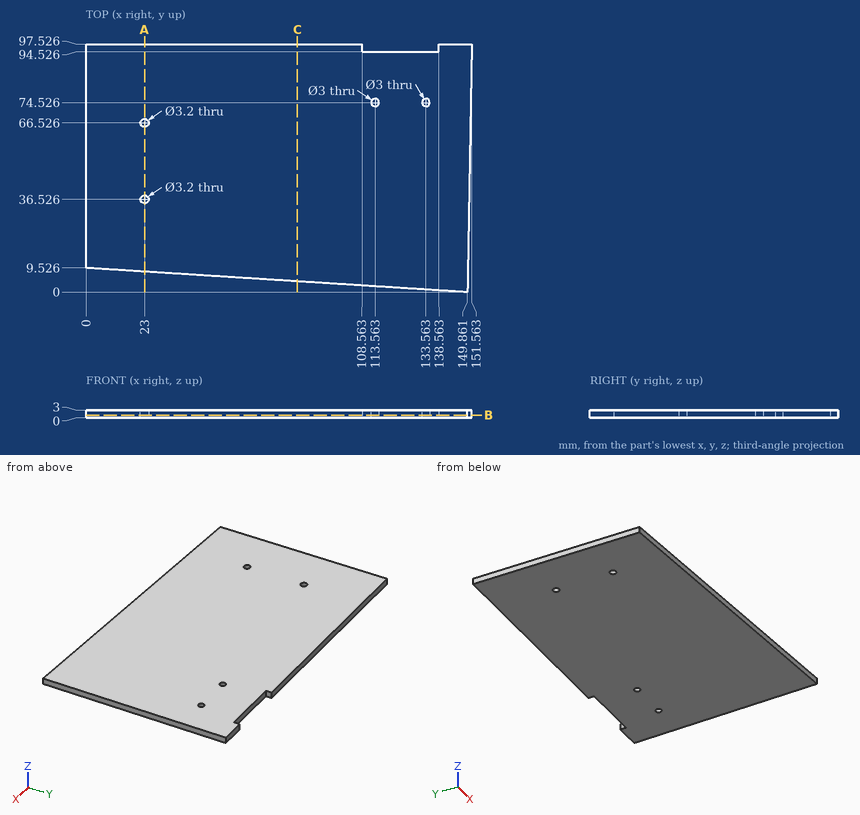
Check sheet for the drawn part. Datum: minimum x, y, z corner. Units: mm. Coordinates: 2 decimals unless noted, no trailing zeros. Order: outer loops, then holes, each group sorted by start corner. A loop starts at its lowest first (then second) coordinate and runs counter-clockwise, first axis right, second up. Notation, with made-up numbers: M 28.5,80.25 L 47.5,80.25 A27 ccw 47.5,99.25 Z; hole C 19,19.5 d10. An arc over 180 degrees is marked long. One line per item, written item: value. Start each with the question number.
Item 1: Sectioned sample at B-B (z = 1.05). Enter the section's corners in (x, y).
Item 2: Sectioned sample at C-C (x = 83). Enter the section's corners in (y, z).
Item 3: Gauge pin test, flat end, axial feed: pin 1 (1 mm diameter, centred on x = 127.5, z = 2, fed in from +Y). Record the tip position at first contact, or that the pin passes through.
Item 4: Sectioned sample at A-A (x = 23). Enter the section's corners in (y, z) (1 decimal).
Item 5: Scan lines: probe 1 along Y at (x, z) = (23, 2) (1 decimal); probe 2 along Y at (x, z) = (132.5, 0.6) (1 decimal); probe 3 along Y at (x, z) = (29.5, 0.35). Record each from-to range of solid material in increasing order.
Conclusion:
1. outline: M 0,9.53 L 149.86,0 L 151.56,97.53 L 138.56,97.53 L 138.56,94.53 L 108.56,94.53 L 108.56,97.53 L 0,97.53 Z; hole C 23,36.53 d3.2; hole C 23,66.53 d3.2; hole C 113.56,74.53 d3; hole C 133.56,74.53 d3
2. outline: M 4.25,0 L 97.53,0 L 97.53,3 L 4.25,3 Z
3. pin 1: stops at y = 94.53
4. outline: M 8.1,0 L 34.9,0 L 34.9,3 L 8.1,3 Z; M 38.1,0 L 64.9,0 L 64.9,3 L 38.1,3 Z; M 68.1,0 L 97.5,0 L 97.5,3 L 68.1,3 Z
5. probe 1: y = 8.1 to 34.9, 38.1 to 64.9, 68.1 to 97.5
5. probe 2: y = 1.1 to 73.5, 75.6 to 94.5
5. probe 3: y = 7.65 to 97.53
